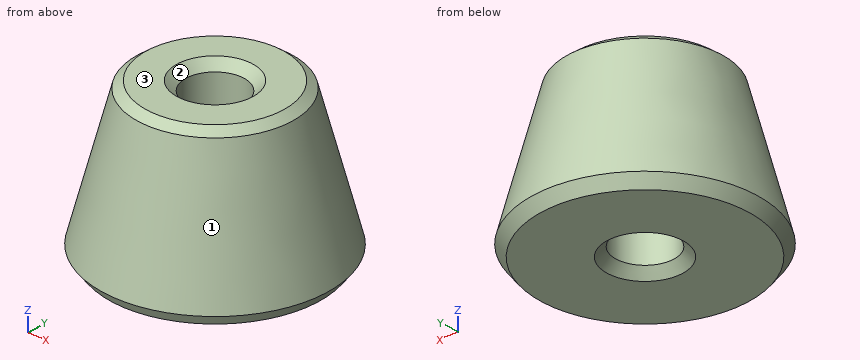
from build123d import *

# Parameters (mm, degrees)
F0_R     = 13
F2_R     = 8.5
F4_R     = 3.275
F5_DEPTH = 25


# Not quite as in the source:
# - a fillet or chamfer that OpenCascade refuses, or shapes differently, is made with other operations: its cross-section is extruded or revolved along the edge and cut away or added


with BuildPart() as f3:
    # F0 (on Top) → F3 section 0
    with BuildSketch(Plane.XY):
        Circle(F0_R)
    # F2 (on offset) → F3 section 1
    with BuildSketch(Plane.XY.offset(17)):
        Circle(F2_R)
    loft()

    # F4 (on face) → F5 (cut)
    with BuildSketch(Plane.XY.offset(17)):
        Circle(F4_R)
    extrude(amount=-F5_DEPTH, mode=Mode.SUBTRACT)

    # F6: chamfer of 1 on 4 edges, made by hand

    # F6_s1 → F6_t2 (revolve, cut)
    with BuildSketch(Plane.XZ):
        Polygon((4.275, 17), (3.275, 16), (3.275, 17), align=None)
    revolve(axis=Axis((0, 0, 17), (0, 0, 1)), mode=Mode.SUBTRACT)

    # F6_s3 → F6_t4 (revolve, cut)
    with BuildSketch(Plane.XZ):
        Polygon((8.6969696164, 16.2558925603), (7.7302643885, 17), (8.5, 17), align=None)
    revolve(axis=Axis((0, 0, 17), (0, 0, 1)), mode=Mode.SUBTRACT)

    # F6_s5 → F6_t6 (revolve, cut)
    with BuildSketch(Plane.XZ):
        Polygon((12.6675578517, 1.2558925603), (11.7008526238, 0), (13, 0), align=None)
    revolve(axis=Axis((0, 0, 0), (0, 0, 1)), mode=Mode.SUBTRACT)

    # F6_s7 → F6_t8 (revolve, cut)
    with BuildSketch(Plane.XZ):
        Polygon((4.275, 0), (3.275, 1), (3.275, 0), align=None)
    revolve(axis=Axis((0, 0, 0), (0, 0, 1)), mode=Mode.SUBTRACT)


solid = f3.part
Read the model definition and answer for the solid it produces. Units are mm, in the model's axes. Face numbers are marked on the shaded views. Round coordinates to 2 decimals unless told otherwise and drop trailing zeros. Loops run counter-clockwise (first coordinate to the right, second up) from the corner with the lowest first, then second, coordinate; pieces in that order, holes last.
Q1. Section B-B on z = 10 is taken. Write down the section's boundary in (x, y) (3 decimals).
Q2. Each of these flat-tipped pins is pushed along its axis until it touches: pin 1 (10 mm diameter, centred on y = 3.5, z = 8, fed in from -X); pin 2 (5 mm diameter, centred on y = -1, z = 10.5, fed in from +X); pin 3 (5 mm diameter, centred on x = 9, z = 6.5, fed in from +Y). Where does it stop, or does it pass through?
Q3. Section A-A on x = 0 is taken. Write down the section's boundary in (y, z) (3 decimals), and give its area (3 significant figures).
Q4. Section C-C on z = 15.25 is taken. Write down the section's boundary in (x, y) (3 decimals), and give its area (3 significant figures).
Q5. Determine the mould class of the marked faces 1, 2 and 3 for opening direction X: released by +X, released by -X, zero draft, split by the parting line, or undercut.
Q6. Consider probe 1 along X at (y, z) = (-1.5, 11.25); probe 2 along Y at (x, z) = (0, 13.25) (3 decimals); probe 3 along Y at (x, z) = (0, 12.75) (3 decimals). Determine where each line is inside the solid, lowest interval first.
Output:
1. outline: circle Ø20.706 at (0, 0); hole circle Ø6.55 at (0, 0)
2. pin 1: stops at x = -12
2. pin 2: stops at x = 10.86
2. pin 3: stops at y = 9.39
3. outline: (-12.668, 1.256) - (-11.701, 0) - (-4.275, 0) - (-3.275, 1) - (-3.275, 16) - (-4.275, 17) - (-7.73, 17) - (-8.697, 16.256) - close; (3.275, 1) - (4.275, 0) - (11.701, 0) - (12.668, 1.256) - (8.697, 16.256) - (7.73, 17) - (4.275, 17) - (3.275, 16) - close
3. area: 250 mm2
4. outline: circle Ø17.926 at (0, 0); hole circle Ø6.55 at (0, 0)
4. area: 219 mm2
5. face 1: split by the parting line
5. face 2: undercut
5. face 3: zero draft
6. probe 1: x = -9.91 to -2.91, 2.91 to 9.91
6. probe 2: y = -9.493 to -3.275, 3.275 to 9.493
6. probe 3: y = -9.625 to -3.275, 3.275 to 9.625
